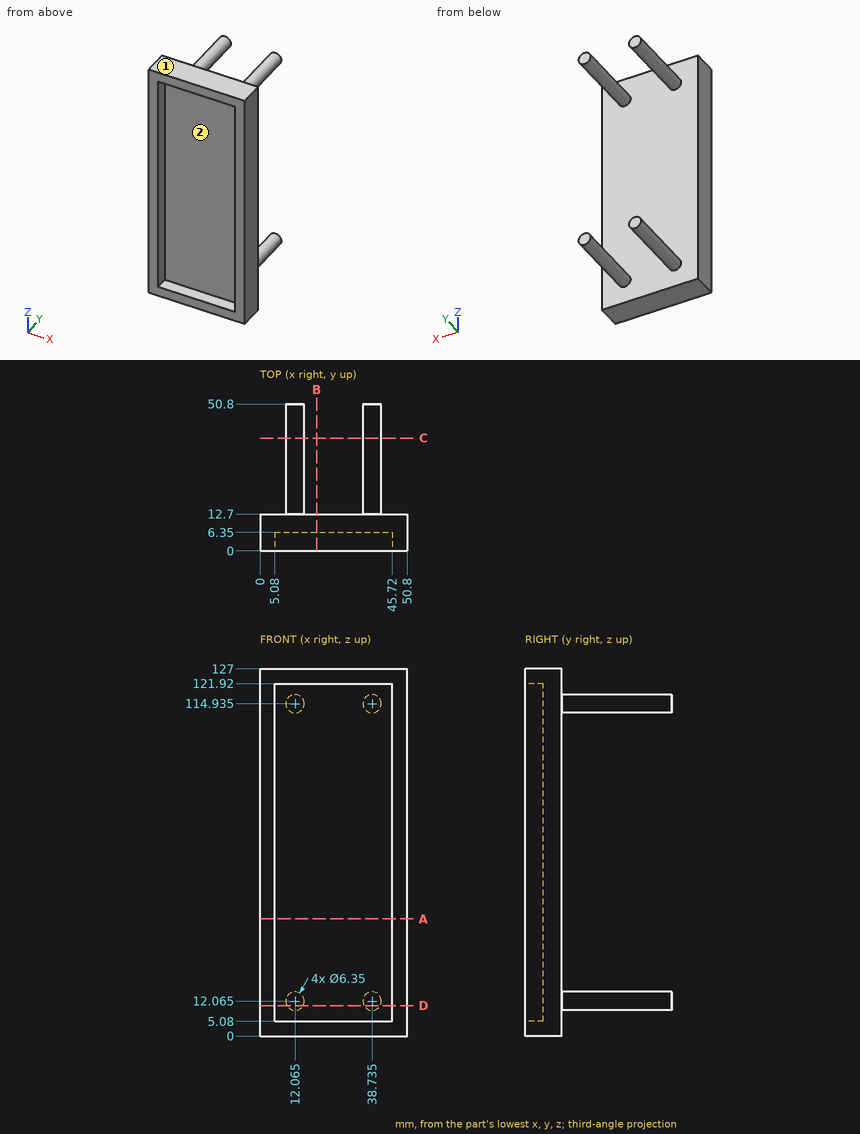
Answer from the drawing. Dimensions are ordinates in mm from the lowest x, y and z of the part. A direction names the side the tool comes from. Coordinates: 2 decimals unless noted, no trailing zeros. Order: outer loops, then holes, each group sorted by start corner. A loop starts at its lowest first (then second) coordinate and runs counter-clockwise, first axis right, second up. Notation, with made-up numbers: (-26.5, 77.5) -> (24.5, 77.5) arc R6 cw to (24.5, 86.5) -> close; hole circle Ø11 at (-5, 24). An arc over 180 degrees is marked (long way). Answer as a JSON object with one key per item and string values.
1) A cutting plane is placed at D-D, the plane z = 10.5. Determine the outline of the cut face in (x, y).
Model answer:
{"outline": "(0, 0) -> (5.08, 0) -> (5.08, 6.35) -> (45.72, 6.35) -> (45.72, 0) -> (50.8, 0) -> (50.8, 12.7) -> (41.5, 12.7) -> (41.5, 50.8) -> (35.97, 50.8) -> (35.97, 12.7) -> (14.83, 12.7) -> (14.83, 50.8) -> (9.3, 50.8) -> (9.3, 12.7) -> (0, 12.7) -> close"}
2) A cutting plane is placed at C-C, the plane y = 39. Determine the outline of the cut face in (x, z) (3 decimals).
Model answer:
{"outline": "circle Ø6.35 at (12.065, 12.065); circle Ø6.35 at (12.065, 114.935); circle Ø6.35 at (38.735, 12.065); circle Ø6.35 at (38.735, 114.935)"}
3) A tool of negligible diameter and unlimited length cuts with its end or side. For the marked faces 1 and 2, from which of +Z, -Z, +X, -X, +Y, -Y can it reach the whole face along a straight path? Write none if from no direction.
Model answer:
{"face 1": "+Z, +X, -X, +Y, -Y", "face 2": "-Y"}
4) A cutting plane is placed at B-B, the plane x = 19.5. Determine the outline of the cut face in (y, z).
Model answer:
{"outline": "(0, 0) -> (12.7, 0) -> (12.7, 127) -> (0, 127) -> (0, 121.92) -> (6.35, 121.92) -> (6.35, 5.08) -> (0, 5.08) -> close"}
5) Consider line 1 along Y through (x, z) = (33, 100.5); line 2 along Y through (x, z) = (47, 38); line 3 along X through (y, z) = (3, 63.5). Determine where each line is inside the solid, lowest interval first. Write a range as from..to.
Model answer:
{"line 1": "y = 6.35..12.7", "line 2": "y = 0..12.7", "line 3": "x = 0..5.08, 45.72..50.8"}
6) A cutting plane is placed at A-A, the plane z = 40.5. Determine the outline of the cut face in (x, y), plus the area to 3 significant figures.
Model answer:
{"outline": "(0, 0) -> (5.08, 0) -> (5.08, 6.35) -> (45.72, 6.35) -> (45.72, 0) -> (50.8, 0) -> (50.8, 12.7) -> (0, 12.7) -> close", "area": "387 mm²"}
7) Each of these flat-tipped pins is pushed along its axis until it touches: pin 1 (2 mm diameter, centred on x = 20.5, z = 18.5, fed in from -Y); pin 2 (12 mm diameter, centred on y = 14, z = 108.5, fed in from -X); pin 3 (8 mm diameter, centred on x = 36.5, y = 37.5, fed in from -Z); pin 4 (1 mm diameter, centred on x = 9.5, z = 55.5, fed in from +Y). Where does it stop, or does it pass through?
Model answer:
{"pin 1": "stops at y = 6.35", "pin 2": "stops at x = 0", "pin 3": "stops at z = 8.89", "pin 4": "stops at y = 12.7"}
